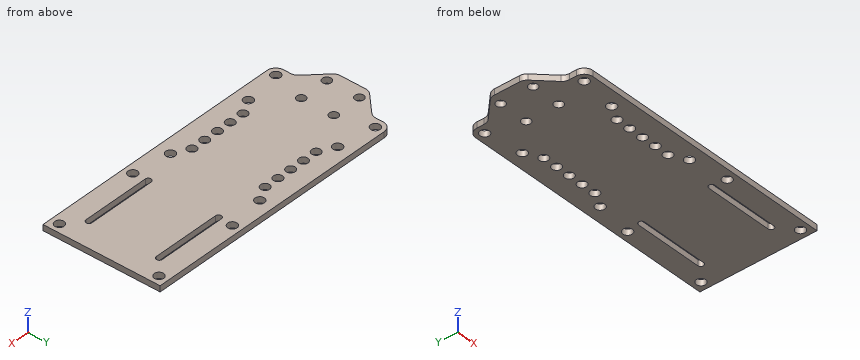
from build123d import *

# Parameters (mm, degrees)
F0_R     = 1.6
F0_R_2   = 1.5
F0_W     = 37.7
F0_H     = 37.7
F0_R_3   = 1.55
F1_DEPTH = 2
F2_R     = 3


with BuildPart() as f1:
    # F0 (on Top) → F1 (new body)
    with BuildSketch(Plane.XY):
        Polygon((-31, -20), (0, -20), (59.73597, -20), (59.73597, 0), (59.73597, 20), (0, 20), (-31, 20), (-31, 13.2831567489), (-38.7195013463, 5.5636554025), (-38.7195013463, -5.5636554025), (-31, -13.2831567489), align=None)
        with Locations((-28, -17)):
            Circle(F0_R, mode=Mode.SUBTRACT)
        with BuildLine():
            ThreePointArc((-33.3597506732, -5.5636554025), (-34.8597506732, -7.0636554025), (-36.3597506732, -5.5636554025))
            ThreePointArc((-36.3597506732, -5.5636554025), (-34.8597506732, -4.0636554025), (-33.3597506732, -5.5636554025))
        make_face(mode=Mode.SUBTRACT)
        with Locations((-24.844666943, -5.5636554025)):
            Circle(F0_R_2, mode=Mode.SUBTRACT)
        with Locations((28, -17)):
            Circle(F0_R, mode=Mode.SUBTRACT)
        with Locations((56.73597, -17)):
            Circle(F0_R, mode=Mode.SUBTRACT)
        with BuildLine():
            Line((27.7028705632, -11), (39.292985, -11))
            Line((39.292985, -11), (50.8830994368, -11))
            ThreePointArc((50.8830994368, -11), (51.8830994368, -12), (50.8830994368, -13))
            Line((50.8830994368, -13), (39.292985, -13))
            Line((39.292985, -13), (27.7028705632, -13))
            ThreePointArc((27.7028705632, -13), (26.7028705632, -12), (27.7028705632, -11))
        make_face(mode=Mode.SUBTRACT)
        with BuildLine():
            ThreePointArc((-33.3597506732, 5.5636554025), (-34.8597506732, 4.0636554025), (-36.3597506732, 5.5636554025))
            ThreePointArc((-36.3597506732, 5.5636554025), (-34.8597506732, 7.0636554025), (-33.3597506732, 5.5636554025))
        make_face(mode=Mode.SUBTRACT)
        with Locations((-24.844666943, 5.5636554025)):
            Circle(F0_R_2, mode=Mode.SUBTRACT)
        Rectangle(F0_W, F0_H, mode=Mode.SUBTRACT)
        with Locations((-28, 17)):
            Circle(F0_R, mode=Mode.SUBTRACT)
        with Locations((28, 17)):
            Circle(F0_R, mode=Mode.SUBTRACT)
        with BuildLine():
            Line((50.8830994368, 11), (39.292985, 11))
            Line((39.292985, 11), (27.7028705632, 11))
            ThreePointArc((27.7028705632, 11), (26.7028705632, 12), (27.7028705632, 13))
            Line((27.7028705632, 13), (39.292985, 13))
            Line((39.292985, 13), (50.8830994368, 13))
            ThreePointArc((50.8830994368, 13), (51.8830994368, 12), (50.8830994368, 11))
        make_face(mode=Mode.SUBTRACT)
        with Locations((56.73597, 17)):
            Circle(F0_R, mode=Mode.SUBTRACT)
        Rectangle(F0_W, F0_H)
        with Locations((-15.25, -15.25)):
            Circle(F0_R, mode=Mode.SUBTRACT)
        with Locations((-10, -12.5)):
            Circle(F0_R_3, mode=Mode.SUBTRACT)
        with Locations((-5, -12.5)):
            Circle(F0_R_3, mode=Mode.SUBTRACT)
        with Locations((0, -12.5)):
            Circle(F0_R_3, mode=Mode.SUBTRACT)
        with Locations((5, -12.5)):
            Circle(F0_R_3, mode=Mode.SUBTRACT)
        with Locations((10, -12.5)):
            Circle(F0_R_3, mode=Mode.SUBTRACT)
        with Locations((15.25, -15.25)):
            Circle(F0_R, mode=Mode.SUBTRACT)
        with Locations((-15.25, 15.25)):
            Circle(F0_R, mode=Mode.SUBTRACT)
        with Locations((-10, 12.5)):
            Circle(F0_R_3, mode=Mode.SUBTRACT)
        with Locations((-5, 12.5)):
            Circle(F0_R_3, mode=Mode.SUBTRACT)
        with Locations((0, 12.5)):
            Circle(F0_R_3, mode=Mode.SUBTRACT)
        with Locations((5, 12.5)):
            Circle(F0_R_3, mode=Mode.SUBTRACT)
        with Locations((10, 12.5)):
            Circle(F0_R_3, mode=Mode.SUBTRACT)
        with Locations((15.25, 15.25)):
            Circle(F0_R, mode=Mode.SUBTRACT)
    extrude(amount=F1_DEPTH)

    # F2
    f2_edges = [f1.edges().sort_by_distance(p)[0] for p in [
        (-31, -20, 1),
        (-31, 20, 1),
        (-31, 13.283157, 1),
        (-38.719501, 5.563655, 1),
        (-38.719501, -5.563655, 1),
        (-31, -13.283157, 1),
    ]]
    fillet(f2_edges, radius=F2_R)


solid = f1.part
Geometry: final body of the model. Coordinates: model frame, mm. Give positions to 0.01 mm unless a question says otherwise; leave off trailing zeros. Loops run counter-clockwise (first coordinate to the right, second up) from the corner with the lowest first, then second, coordinate; pieces in that order, holes last. Notation, with made-up numbers: M 23,-37.5 L 50,-37.5 A25 ccw 50,-10.5 Z; hole C 7.25,69 d10. An arc over 180 degrees is marked long. Put each result on its own line as item: value. Start each with the question number.
1) Cut plane D-D (z = 0.5). Give the number of separate pieces and of enclosed holes in the cut face, then the cut area to 3 significant figures.
2) Ray query, line 1 along Y through (x, z) = (5, 0.9); line 2 along Y through (x, z) = (15.25, 0.7); line 3 along Y through (x, z) = (29, 0.6). Return the intervals inside material, ascending.
3) Cut plane B-B (x = -15.25). Output: boundary loops of the cut face in (y, z).
4) Cut plane A-A (x = 37). Output: boundary loops of the cut face in (y, z), then the cut area to 3 significant figures.
5) Cut plane C-C (y = 8). Output: boundary loops of the cut face in (x, z).
6) Contact query for flat-ended pins moving along their axis: pin 1 (5 mm diameter, centred on x = 0, y = 12.5, fed in from +Z); pin 2 (0.6 mm diameter, centred on y = -16, z = 1, fed in from -X). Output: stop coordinate, or through.
Verdict:
1. separate pieces: 1
1. enclosed holes: 26
1. area: 3,490 mm2
2. line 1: -20 to -14.05, -10.95 to 10.95, 14.05 to 20
2. line 2: -20 to -16.85, -13.65 to 13.65, 16.85 to 20
2. line 3: -20 to -18.25, -15.75 to -13, -11 to 11, 13 to 15.75, 18.25 to 20
3. outline: M -20,0 L -16.85,0 L -16.85,2 L -20,2 Z; M -13.65,0 L 13.65,0 L 13.65,2 L -13.65,2 Z; M 16.85,0 L 20,0 L 20,2 L 16.85,2 Z
4. outline: M -20,0 L -13,0 L -13,2 L -20,2 Z; M -11,0 L 11,0 L 11,2 L -11,2 Z; M 13,0 L 20,0 L 20,2 L 13,2 Z
4. area: 72.0 mm2
5. outline: M -36.28,0 L 59.74,0 L 59.74,2 L -36.28,2 Z
6. pin 1: z = 2
6. pin 2: x = -31
